Can you work these out from the model? Positions are in its coordinate system, mm. Face numbers are marked on the shaded views. A direction names the side the tool comes from. Give positions to 0.01 mm unless a question says otherwise; leave off trailing zeros. Order: outer loops, then holes, each group sorted by start corner. A loop starts at its lowest first (then second) coordinate and runs counter-clockwise, first axis right, second up.
Item 1: I want a section at A-A, the plane y = 0. Write out the boundary of the cut face in (x, z).
Item 2: I'm going to push flat-ended pins straight in: pin 1 Ø2 at (x, z) = (2, -59.5) entering from -Y; pin 2 Ø3 at (y, z) = (3, -42) entering from -X; pin 3 Ø1 at (y, z) = (-6, -73) entering from +X; pin 4 Ø2 at (y, z) = (0.5, -23.5) entering from -X. Where does each tip first touch, or does it pass through?
Item 3: I want a section at C-C, the plane z = -62. Write out the boundary of the cut face in (x, y).
Item 4: If I drill on line 1 along Z through (x, y) = (6.5, 0); line 2 along X through (y, z) = (0.25, -59); line 3 along Y through (x, z) = (-1.5, -46), over which ranges is the centre line in solid material (lowest first)?
Item 5: Which directions (+Z, -Z, +X, -X, +Y, -Y) give clear straight access to the entire face, cutting with the end or side of a thin tool? Please do the marked faces 1 and 2.
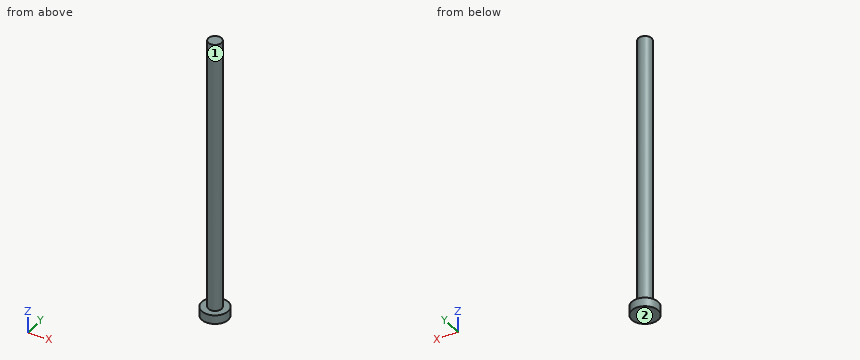
Autodesk Inventor part; units mm, degrees
ref_plane "YZ Plane" through (0, 0, 0) normal (1, 0, 0) x (0, 1, 0)
ref_plane "XZ Plane" through (0, 0, 0) normal (0, 1, 0) x (-1, 0, 0)
ref_plane "XY Plane" through (0, 0, 0) normal (0, 0, 1) x (1, 0, 0)
sketch "Sketch1" plane through (0, 0, 0) normal (0, 0, 1) x (1, 0, 0)
  circle A0 centre (0, 0) radius 3.81
  dimension "d0" = 7.62
extrude "Extrusion1" add sketch "Sketch1" against normal blind 157.48
sketch "Sketch2" plane through (0, 0, -157.48) normal (0, 0, -1) x (-1, 0, 0)
  circle A0 centre (0, 0) radius 7.62
  circle A1 centre (0, 0) radius 3.81
  dimension "d3" = 15.24
extrude "Extrusion2" add sketch "Sketch2" against normal blind 5.08
sketch "Sketch3" plane through (0, 0, 0) normal (0, 0, 1) x (1, 0, 0)
  circle A0 centre (0, 0) radius 3.81
extrude "Extrusion3" add sketch "Sketch3" along normal blind 5.08
properties part number "roller pin"
Results list:
1. outline: (-7.62, -157.48) - (7.62, -157.48) - (7.62, -152.4) - (3.81, -152.4) - (3.81, 5.08) - (-3.81, 5.08) - (-3.81, -152.4) - (-7.62, -152.4) - close
2. pin 1: stops at y = -3.68
2. pin 2: stops at x = -3.5
2. pin 3: passes through
2. pin 4: stops at x = -3.81
3. outline: circle Ø7.62 at (0, 0)
4. line 1: z = -157.48 to -152.4
4. line 2: x = -3.8 to 3.8
4. line 3: y = -3.5 to 3.5
5. face 1: +Z
5. face 2: -Z, +X, -X, +Y, -Y
